Work out the finished part from the listing and answer in its coordinate system (mm). Face numbers are marked on the shaded views. A direction names the side the tool comes from. Coordinates: 2 decimals unless noted, no trailing zeros. Write each loop counter-clockwise with the first axis right and the second up, starting at its lowest first coordinate (ties: lowest second). Pieces come first, ordered by that corner, then holes. Notation, with made-up numbers: (-3.75, -36) - (44.25, -36) arc R22 cw to (44.25, -2) - close; hole circle Ø11 at (-40, 71.25). An arc over 180 degrees is marked (long way). One line per item, written item: value.
```python
from build123d import *

# Parameters (mm, degrees)
BOSS_EXTRUDE1_DEPTH       = 23
CUT_EXTRUDE1_REACH        = 120.347
SKETCH2_R                 = 1.25
CUT_EXTRUDE2_REACH        = 114.739
SKETCH3_R                 = 1.75
BOSS_EXTRUDE2_START       = -11.4
BOSS_EXTRUDE2_DEPTH       = 11.5
LPATTERN1_COUNT           = 2
LPATTERN1_PITCH           = 66
DRAFT1_ANGLE              = 4
MIRROR1_START             = -11.4
MIRROR1_COPY_1_DEPTH      = 11.5
DRAFT1_OF_MIRROR1_2_ANGLE = 4
SKETCH5_W                 = 5
SKETCH5_H                 = 6
CUT_EXTRUDE3_DEPTH        = 11


with BuildPart() as part:
    # Sketch1 → Boss-Extrude1 (new, symmetric)
    with BuildSketch(Plane.XY):
        Polygon((-62, 0), (49, 0), (49, -34), (43, -34), (43, -6), (-56, -6), (-56, -34), (-62, -34), align=None)
    extrude(amount=BOSS_EXTRUDE1_DEPTH, both=True)

    # Sketch2 → Cut-Extrude1 (cut, up to next)
    with BuildSketch(Plane.ZY.offset(62), mode=Mode.PRIVATE) as cut_extrude1_sk1:
        with Locations((-6.328605692, -16.671394308)):
            Circle(SKETCH2_R)
    cut_extrude1_tool1 = extrude(cut_extrude1_sk1.sketch, amount=-CUT_EXTRUDE1_REACH, mode=Mode.PRIVATE) & part.part
    # Sketch2 → Cut-Extrude1 (cut, up to next)
    with BuildSketch(Plane.ZY.offset(62), mode=Mode.PRIVATE) as cut_extrude1_sk2:
        with Locations((6.328605692, -16.671394308)):
            Circle(SKETCH2_R)
    cut_extrude1_tool2 = extrude(cut_extrude1_sk2.sketch, amount=-CUT_EXTRUDE1_REACH, mode=Mode.PRIVATE) & part.part
    # Sketch2 → Cut-Extrude1 (cut, up to next)
    with BuildSketch(Plane.ZY.offset(62), mode=Mode.PRIVATE) as cut_extrude1_sk3:
        with Locations((6.328605692, -29.328605692)):
            Circle(SKETCH2_R)
    cut_extrude1_tool3 = extrude(cut_extrude1_sk3.sketch, amount=-CUT_EXTRUDE1_REACH, mode=Mode.PRIVATE) & part.part
    # Sketch2 → Cut-Extrude1 (cut, up to next)
    with BuildSketch(Plane.ZY.offset(62), mode=Mode.PRIVATE) as cut_extrude1_sk4:
        with Locations((-6.328605692, -29.328605692)):
            Circle(SKETCH2_R)
    cut_extrude1_tool4 = extrude(cut_extrude1_sk4.sketch, amount=-CUT_EXTRUDE1_REACH, mode=Mode.PRIVATE) & part.part
    # Sketch2 → Cut-Extrude1 (cut, up to next)
    with BuildSketch(Plane.ZY.offset(62), mode=Mode.PRIVATE) as cut_extrude1_sk5:
        Polygon((-5, -20.113248654), (-5, -25.886751346), (0, -28.773502692), (5, -25.886751346), (5, -20.113248654), (0, -17.226497308), align=None)
    cut_extrude1_tool5 = extrude(cut_extrude1_sk5.sketch, amount=-CUT_EXTRUDE1_REACH, mode=Mode.PRIVATE) & part.part
    add(cut_extrude1_tool1.solids().sort_by_distance((-62, -16.671394, -6.328606))[0], mode=Mode.SUBTRACT)
    add(cut_extrude1_tool2.solids().sort_by_distance((-62, -16.671394, 6.328606))[0], mode=Mode.SUBTRACT)
    add(cut_extrude1_tool3.solids().sort_by_distance((-62, -29.328606, 6.328606))[0], mode=Mode.SUBTRACT)
    add(cut_extrude1_tool4.solids().sort_by_distance((-62, -29.328606, -6.328606))[0], mode=Mode.SUBTRACT)
    add(cut_extrude1_tool5.solids().sort_by_distance((-62, -23, 0))[0], mode=Mode.SUBTRACT)

    # Sketch3 → Cut-Extrude2 (cut, up to next)
    with BuildSketch(Plane.ZY.offset(-43), mode=Mode.PRIVATE) as cut_extrude2_sk1:
        with Locations((0, -23)):
            Circle(SKETCH3_R)
    cut_extrude2_tool1 = extrude(cut_extrude2_sk1.sketch, amount=-CUT_EXTRUDE2_REACH, mode=Mode.PRIVATE) & part.part
    add(cut_extrude2_tool1.solids().sort_by_distance((43, -23, 0))[0], mode=Mode.SUBTRACT)

    # Sketch4 → Boss-Extrude2 (add)
    with BuildSketch(Plane(origin=(0, 0, 0), x_dir=(-1, 0, 0), z_dir=(0, 0, -1)).offset(BOSS_EXTRUDE2_START)):
        with BuildLine():
            Line((28.9, -16.213224045), (28.9, -6))
            Line((28.9, -6), (26.6, -6))
            Line((26.6, -6), (26.6, -21.5))
            ThreePointArc((26.6, -21.5), (34.4134809, -24.276355191), (30.103703704, -17.192256629))
            ThreePointArc((30.103703704, -17.192256629), (29.269010184, -16.989015158), (28.9, -16.213224045))
        make_face()
    boss_extrude2 = extrude(amount=-BOSS_EXTRUDE2_DEPTH)

    # LPattern1: Boss-Extrude2 ×2
    with Locations(*[(i * LPATTERN1_PITCH, 0, 0) for i in range(1, LPATTERN1_COUNT)]):
        add(boss_extrude2)

    # Draft1
    draft1_faces = [part.faces().sort_by_distance(p)[0] for p in [
        (36.075013094, -18.535245668, 22.9),
        (-29.924986906, -18.535245668, 22.9),
    ]]
    draft(draft1_faces, Plane.ZX.offset(-21.5), DRAFT1_ANGLE)

    # Mirror1: Boss-Extrude2 across plane
    add(boss_extrude2.mirror(Plane.XY))

    # Mirror1 copy 1 sketch → Mirror1 copy 1 (add)
    with BuildSketch(Plane(origin=(66, 0, 0), x_dir=(-1, 0, 0), z_dir=(0, 0, 1)).offset(MIRROR1_START)):
        with BuildLine():
            Line((28.9, 16.213224045), (28.9, 6))
            Line((28.9, 6), (26.6, 6))
            Line((26.6, 6), (26.6, 21.5))
            ThreePointArc((26.6, 21.5), (34.4134809, 24.276355191), (30.103703704, 17.192256629))
            ThreePointArc((30.103703704, 17.192256629), (29.269010184, 16.989015158), (28.9, 16.213224045))
        make_face()
    extrude(amount=-MIRROR1_COPY_1_DEPTH)

    # Draft1 of Mirror1 2
    draft1_of_mirror1_2_faces = [part.faces().sort_by_distance(p)[0] for p in [
        (36.075013094, -18.535245668, -22.9),
        (-29.924986906, -18.535245668, -22.9),
    ]]
    draft(draft1_of_mirror1_2_faces, Plane(origin=(0, -21.5, 0), x_dir=(0, 0, -1), z_dir=(0, 1, 0)), DRAFT1_OF_MIRROR1_2_ANGLE)

    # Sketch5 → Cut-Extrude3 (cut)
    with BuildSketch(Plane.XY.offset(23)):
        with Locations((-35.2, -3)):
            Rectangle(SKETCH5_W, SKETCH5_H)
        with Locations((30.8, -3)):
            Rectangle(SKETCH5_W, SKETCH5_H)
    extrude(amount=-CUT_EXTRUDE3_DEPTH, mode=Mode.SUBTRACT)


solid = part.part
```
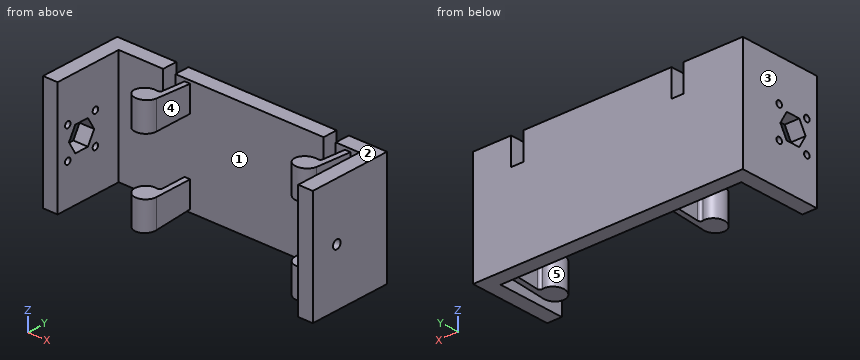
Item 1: Section A-A, the plane y = -12 is taken. Determine the outline of the cut face in (x, z).
Evaluation:
outline: (-62, -23) - (-56, -23) - (-56, 23) - (-62, 23) - close; (-28.9, -22.24) - (-26.6, -22.24) - (-26.6, -11.4) - (-28.9, -11.4) - close; (-28.9, 11.4) - (-26.6, 11.4) - (-26.6, 22.24) - (-28.9, 22.24) - close; (37.1, -22.24) - (39.4, -22.24) - (39.4, -11.4) - (37.1, -11.4) - close; (37.1, 11.4) - (39.4, 11.4) - (39.4, 22.24) - (37.1, 22.24) - close; (43, -23) - (49, -23) - (49, 23) - (43, 23) - close
Item 2: Section D-D, the plane y = -23 is taken. Give the number of separate pieces and of enclosed holes in the cut face, then the cut area to 3 significant figures.
Evaluation:
separate pieces: 8
enclosed holes: 0
area: 855 mm2
Item 3: Which of the six approach directions +Z, -Z, +X, -X, +Y, -Y give full straight-line access (tool end or side, diameter ignored) to the marked faces 4 and 5?
Evaluation:
face 4: +Z, -Z, -Y
face 5: +Z, -Z
Item 4: Section B-B, the plane z = 16.5 is taken. Determine the outline of the cut face in (x, y).
Evaluation:
outline: (-62, -34) - (-56, -34) - (-56, -6) - (-37.7, -6) - (-37.7, 0) - (-62, 0) - close; (-32.7, -6) - (-28.9, -6) - (-28.9, -16.21) arc R1 cw to (-30.1, -17.19) arc R4.4 ccw (long way) to (-26.6, -21.5) - (-26.6, -6) - (28.3, -6) - (28.3, 0) - (-32.7, 0) - close; (33.3, -6) - (37.1, -6) - (37.1, -16.21) arc R1 cw to (35.9, -17.19) arc R4.4 ccw (long way) to (39.4, -21.5) - (39.4, -6) - (43, -6) - (43, -34) - (49, -34) - (49, 0) - (33.3, 0) - close
Item 5: Section C-C, the plane z = 10 is taken. Determine the outline of the cut face in (x, y), then the cut area to 3 significant figures.
Evaluation:
outline: (-62, -34) - (-56, -34) - (-56, -6) - (43, -6) - (43, -34) - (49, -34) - (49, 0) - (-62, 0) - close
area: 1,000 mm2
Item 6: Given pin 1 (10 mm diameter, centred on x = -33.5, y = -20, fed in from -Z); pin 2 (2 mm diameter, centred on y = -16.67, z = -6.33, fed in from -X); pin 3 (4.5 mm diameter, centred on x = -60, y = -23.5, fed in from -Z), each flat-ended and moving along its own axis, determine where each tip first touches the part or whether it passes through.
Evaluation:
pin 1: stops at z = -23.14
pin 2: stops at x = 43
pin 3: stops at z = -23
Item 7: Determine the mould class of the marked faces 1, 2 and 3 for opening direction X: +X half, -X half, draft (parallel to the pull), parting line (faces both ways), or undercut.
Evaluation:
face 1: undercut
face 2: draft
face 3: -X half
Item 8: Consider probe 1 along X at (y, z) = (-8, 14); probe 2 along X at (y, z) = (-16, 1.5); probe 3 along X at (y, z) = (-22, -17.5). Determine where each line is inside the solid, lowest interval first.
Evaluation:
probe 1: x = -62 to -56, -28.9 to -26.6, 37.1 to 39.4, 43 to 49
probe 2: x = -62 to -56, 43 to 49
probe 3: x = -62 to -56, -35.37 to -26.63, 30.63 to 39.37, 43 to 49
